For this review, take the finished solid that the model builds, in its own axes (mm). A direction names the side the tool comes from. Round coordinates to 2 decimals unless told otherwise and drop trailing zeros. Order: outer loops, then holes, each group sorted by start corner. A loop starts at its lowest first (then second) coordinate and runs counter-clockwise, first axis right, second up. Notation, with made-up numbers: (-26.5, 89) -> (-17.5, 89) arc R6 cw to (-17.5, 99) -> close; hole circle Ø1 at (-17, 21.5). An arc over 180 degrees is marked (long way). Answer in a Markdown table with one row per item.
```python
from build123d import *

# Parameters (mm, degrees)
SKETCH1_R           = 5
BOSS_EXTRUDE1_DEPTH = 1.25
SKETCH2_R           = 1.25
BOSS_EXTRUDE2_DEPTH = 15
BOSS_EXTRUDE3_DEPTH = 1


with BuildPart() as part:
    # Sketch1 → Boss-Extrude1 (new, symmetric)
    with BuildSketch(Plane.XY):
        Circle(SKETCH1_R)
    extrude(amount=BOSS_EXTRUDE1_DEPTH, both=True)

    # Sketch2 → Boss-Extrude2 (add)
    with BuildSketch(Plane.XY.offset(1.25)):
        Circle(SKETCH2_R)
    extrude(amount=BOSS_EXTRUDE2_DEPTH)

    # Sketch4 → Boss-Extrude3 (add)
    # profile 1 of 2: a face of its own
    with BuildSketch(Plane(origin=(0, 0, -1.25), x_dir=(-1, 0, 0), z_dir=(0, 0, -1))):
        Polygon((-1.553943212, 1.601672339), (-0.973370295, 1.601672339), (-0.973370295, -1.538327661), (-1.255165167, -1.538327661), (-1.255165167, 1.279621057), (-1.73824209, 1.279621057), align=None)
    # profile 2 of 2: a face of its own
    with BuildSketch(Plane(origin=(0, 0, -1.25), x_dir=(-1, 0, 0), z_dir=(0, 0, -1))):
        with BuildLine():
            Line((1.643296371, 1.68218516), (1.860303583, 1.511724423))
            Line((1.860303583, 1.511724423), (1.030644128, 0.243018493))
            add(Edge.make_bspline(
                [(1.030644128, 0.243018493), (1.085881462, 0.251822928), (1.193628128, 0.268996974), (1.302690105, 0.271830102), (1.355840442, 0.273210801)],
                knots=[0, 0, 0, 0, 1.025318673, 2, 2, 2, 2], degree=3))
            add(Edge.make_bspline(
                [(1.355840442, 0.273210801), (1.387754053, 0.272353032), (1.450575046, 0.27066454), (1.542807435, 0.257670457), (1.631435223, 0.23719307), (1.716091069, 0.207343104), (1.79707883, 0.16921242), (1.874863266, 0.123512976), (1.947982212, 0.067885023), (2.01737727, 0.005744463), (2.080381009, -0.063081632), (2.136161813, -0.13611026), (2.183016706, -0.213265336), (2.221032167, -0.294507781), (2.250552544, -0.379712363), (2.272072888, -0.468770065), (2.284794009, -0.561742299), (2.286521449, -0.624971291), (2.287398935, -0.65708968)],
                knots=[0, 0, 0, 0, 1.04369286, 2.054478336, 3.041073146, 4.015093852, 4.984733326, 5.965804835, 6.960378782, 7.985147595, 9.009457201, 10.008161701, 10.986880575, 11.956520048, 12.937015923, 13.931873656, 14.949455224, 16, 16, 16, 16], degree=3))
            add(Edge.make_bspline(
                [(2.287398935, -0.65708968), (2.286122207, -0.701031472), (2.283609908, -0.787498518), (2.258576216, -0.913436478), (2.219676421, -1.033413649), (2.164073724, -1.145514494), (2.095009529, -1.249585371), (2.010787917, -1.341798617), (1.914395759, -1.424039736), (1.805404746, -1.492811674), (1.68810963, -1.548975554), (1.564885266, -1.5893158), (1.436928341, -1.614151827), (1.350080778, -1.617265453), (1.306148935, -1.618840481)],
                knots=[0, 0, 0, 0, 1.031375318, 2.029502543, 3.004789286, 3.987476834, 4.960371455, 5.9300674, 6.912260825, 7.929083631, 8.949397511, 9.960523116, 10.96833055, 12, 12, 12, 12], degree=3))
            add(Edge.make_bspline(
                [(1.306148935, -1.618840481), (1.263896467, -1.617469462), (1.180201724, -1.614753714), (1.057084303, -1.590561416), (0.938784339, -1.5513499), (0.826130666, -1.497329091), (0.721774459, -1.429094304), (0.628412717, -1.346949859), (0.546510953, -1.252651654), (0.478350865, -1.146214313), (0.424290174, -1.031837609), (0.383748355, -0.912573988), (0.360067154, -0.788858005), (0.356757992, -0.704992069), (0.355091243, -0.662750738)],
                knots=[0, 0, 0, 0, 1.012016664, 2.004627821, 2.994792927, 3.992885782, 4.990978636, 5.973936114, 6.964471063, 7.975201453, 8.993600317, 9.990122807, 10.98767138, 12, 12, 12, 12], degree=3))
            add(Edge.make_bspline(
                [(0.355091243, -0.662750738), (0.356151168, -0.630413597), (0.358315332, -0.564387335), (0.37342626, -0.464388179), (0.397707247, -0.362068065), (0.424899868, -0.275265732), (0.453631415, -0.204156823), (0.477542551, -0.146826263), (0.507304364, -0.087829186), (0.539039341, -0.025142553), (0.575604074, 0.039618093), (0.615361543, 0.107535099), (0.659410944, 0.177528325), (0.690290747, 0.225026832), (0.70607682, 0.249308557)],
                knots=[0, 0, 0, 0, 1.173818275, 2.396712641, 3.66331629, 4.989737886, 5.693666774, 6.447286557, 7.243889047, 8.091586357, 8.998013824, 9.943181721, 10.948533338, 12, 12, 12, 12], degree=3))
            Line((0.70607682, 0.249308557), (1.643296371, 1.68218516))
        make_face()
        with BuildLine():
            add(Edge.make_bspline(
                [(1.296713839, -0.048840481), (1.272793997, -0.049538498), (1.226071596, -0.050901926), (1.157523229, -0.058819438), (1.092647912, -0.073729114), (1.030586141, -0.092718337), (0.972498202, -0.11882794), (0.917961928, -0.150543554), (0.866766425, -0.187883696), (0.819447924, -0.230319371), (0.776546855, -0.276780635), (0.739601497, -0.32654472), (0.70773283, -0.37841232), (0.681821712, -0.432816805), (0.661644901, -0.489737379), (0.647049956, -0.548912248), (0.638927448, -0.610738226), (0.637576143, -0.652663957), (0.636886115, -0.674072853)],
                knots=[0, 0, 0, 0, 1.129588631, 2.206414736, 3.251139165, 4.268635594, 5.265702196, 6.250456724, 7.242448911, 8.251968645, 9.246821453, 10.222880186, 11.173611482, 12.116736599, 13.062300278, 14.020270554, 14.989073742, 16, 16, 16, 16], degree=3))
            add(Edge.make_bspline(
                [(0.636886115, -0.674072853), (0.637448051, -0.695290264), (0.638549923, -0.736894447), (0.648555147, -0.798204454), (0.66383805, -0.857204972), (0.686572005, -0.913591834), (0.713689841, -0.968224531), (0.749490618, -1.019124187), (0.789159392, -1.069382193), (0.83657692, -1.115137799), (0.88746588, -1.15771317), (0.941833816, -1.194926883), (0.998497323, -1.22676305), (1.058221399, -1.251713578), (1.120158692, -1.272190224), (1.184825246, -1.286599665), (1.252266037, -1.294746194), (1.29795029, -1.296099259), (1.321245089, -1.296789199)],
                knots=[0, 0, 0, 0, 0.989467248, 1.94019797, 2.891935182, 3.827694429, 4.772920941, 5.730924762, 6.725747692, 7.756678648, 8.79901574, 9.819492441, 10.826891316, 11.826466727, 12.835195252, 13.867842842, 14.912794438, 16, 16, 16, 16], degree=3))
            add(Edge.make_bspline(
                [(1.321245089, -1.296789199), (1.344539851, -1.296099205), (1.390224029, -1.294746034), (1.457665362, -1.286600274), (1.522329911, -1.27218799), (1.584274493, -1.251721676), (1.643971662, -1.226733009), (1.700585612, -1.195124944), (1.754439388, -1.157484313), (1.805361754, -1.115210557), (1.852581916, -1.06912177), (1.893202103, -1.019572819), (1.92790649, -0.967813153), (1.956107446, -0.913807046), (1.978591005, -0.857170877), (1.993951407, -0.798213588), (2.003935969, -0.736892056), (2.00504068, -0.695289456), (2.005604064, -0.674072853)],
                knots=[0, 0, 0, 0, 1.087397944, 2.132534446, 3.165364764, 4.174271784, 5.174024072, 6.181601208, 7.194203697, 8.236725232, 9.267838612, 10.269026844, 11.221737037, 12.171628256, 13.107553087, 14.05945871, 15.010357665, 16, 16, 16, 16], degree=3))
            add(Edge.make_bspline(
                [(2.005604064, -0.674072853), (2.005110372, -0.652636027), (2.004141416, -0.61056251), (1.993181965, -0.548939904), (1.977982236, -0.489436719), (1.955030603, -0.432426925), (1.925212674, -0.378135493), (1.888893274, -0.326288171), (1.846877768, -0.276487459), (1.798344547, -0.230228254), (1.745511594, -0.18793059), (1.689336469, -0.150591902), (1.630566459, -0.11907978), (1.56926115, -0.092787123), (1.504718107, -0.073813023), (1.437979346, -0.058872685), (1.368191282, -0.050922189), (1.320843125, -0.049543222), (1.296713839, -0.048840481)],
                knots=[0, 0, 0, 0, 0.978206639, 1.919901502, 2.851605144, 3.780102724, 4.718870031, 5.675451981, 6.667674623, 7.690630536, 8.733308323, 9.756129687, 10.767539656, 11.776269907, 12.797430371, 13.836405707, 14.897401972, 16, 16, 16, 16], degree=3))
        make_face(mode=Mode.SUBTRACT)
    extrude(amount=BOSS_EXTRUDE3_DEPTH)


solid = part.part
```
Q1. Take a section at C-C, the plane y = 4.5. Write out the cut boundary in (x, z).
Answer key:
| item | result |
|---|---|
| outline | (-2.18, -1.25) -> (2.18, -1.25) -> (2.18, 1.25) -> (-2.18, 1.25) -> close |
Q2. Tool access review of faces 1 (the face through (0, 0, 16.25)), 2 (the face through (-0.27, -1.22, 8.64)), 3 (the face through (1.255, 0, -2)), 4 (the face through (0.973, 0, -2)): name each direction out of +Z, -Z, +X, -X, +Y, -Y from which nothing blocks a thin tool from reaching the whole face with its end or side.
Answer key:
| item | result |
|---|---|
| face 1 | +Z, +X, -X, +Y, -Y |
| face 2 | +Z |
| face 3 | -Z, +X, -Y |
| face 4 | -Z, +Y, -Y |
Q3. Take a section at B-B, the plane z = 12. Write out the cut boundary in (x, y).
Answer key:
| item | result |
|---|---|
| outline | circle Ø2.5 at (0, 0) |
Q4. Take a section at A-A, the plane x = 0. Write out the cut boundary in (y, z).
Answer key:
| item | result |
|---|---|
| outline | (-5, -1.25) -> (5, -1.25) -> (5, 1.25) -> (1.25, 1.25) -> (1.25, 16.25) -> (-1.25, 16.25) -> (-1.25, 1.25) -> (-5, 1.25) -> close |
Q5. Clearance check with flat-ended pins moving along their axes: pin 1 Ø0.8 at (y, z) = (-0.5, -1.5) entering from -X; pin 2 Ø3 at (x, z) = (-1.5, 7) entering from +Y; pin 3 Ø5 at (y, z) = (-1.5, 8.5) entering from -X. State where each tip first meets the part, or that it passes through.
Answer key:
| item | result |
|---|---|
| pin 1 | stops at x = -5 |
| pin 2 | stops at y = 1.25 |
| pin 3 | stops at x = -1.25 |
Q6. To check wall thickness, follow probe 1 along Z at (x, y) = (4.5, 0); probe 2 along X at (y, z) = (-1, 7.25); probe 3 along Y at (x, z) = (2, -0.5). State the ranges of each line that lie inside material, in increasing order.
Answer key:
| item | result |
|---|---|
| probe 1 | z = -1.25 to 1.25 |
| probe 2 | x = -0.75 to 0.75 |
| probe 3 | y = -4.58 to 4.58 |
Q7. Take a section at D-D, the plane x = -2.5. Write out the cut boundary in (y, z).
Answer key:
| item | result |
|---|---|
| outline | (-4.33, -1.25) -> (4.33, -1.25) -> (4.33, 1.25) -> (-4.33, 1.25) -> close |
Q8. The part is to be moulded in two halves that separate along X. For faces 5 (the face through (1, -1, 1.25)), 6 (the face through (-1.17, 0.96, -1.74)), 7 (the face through (-1.08, -4.88, 0.02)), say which applies: +X half, -X half, draft (parallel to the pull), parting line (faces both ways), or undercut.
Answer key:
| item | result |
|---|---|
| face 5 | draft |
| face 6 | undercut |
| face 7 | parting line |
